Read the model definition and answer for the solid it produces. Units are mm, in the model's axes. A direction names the side the tool comes from. Coordinates: 2 decimals unless noted, no trailing zeros. Loops run counter-clockwise (first coordinate to the right, second up) from the corner with the lowest first, then second, coordinate; pieces in that order, holes last. Notation, with made-up numbers: (-14.5, 28.5) -> (16.5, 28.5) arc R28 cw to (16.5, 49.5) -> close; hole circle Ø9 at (54, 28). An arc over 180 degrees is marked (long way). Answer as a JSON object with one key per item and string values. Group by question number.
Q1. The part is cut by section B-B on x = 101.5. Write down the section's boundary in (y, z).
Q2. The part is cut by section A-A on y = 34. Write down the section's boundary in (x, z).
Q3. Each of these flat-tipped pins is pushed along its axis until it touches: P1, Ø2.5, axis at x = 83, y = 49, coming from the +Z side; P2, Ø1.5, axis at y = 2, z = 1.5, coming from the +X side; P3, Ø1.5, axis at y = 64, z = 1.5, coming from the +X side; P4, Ø0.9, axis at y = 14.5, z = 2, coming from the -X side. Where does it stop, or does it pass through?
Q4. Determine the mould class of faces 5 (the flat face through (76, 33, 3)), 6 (the flat face through (126, 13, 1)), 7 (the cylindrical face through (83.69, 47.67, 1.52)) for opening direction X: released by +X, released by -X, zero draft, split by the parting line, or undercut.
Q5. Straight lines are drawn through the part: line 1 along X through (y, z) = (36.5, 2); line 2 along Y through (x, z) = (114, 1.9); line 3 along X through (y, z) = (9, 2.8). For each, find the intervals that lie inside material, in ascending order. Write a range as [from, to].
Q6. For faces 1 (the flat face through (123, 33, 1)), 2 (the flat face through (123, 1, 1)), 3 (the flat face through (43, 64, 1)), 4 (the flat face through (99, 49, 2)), determine the directions among +Z, -Z, +X, -X, +Y, -Y from which every point of the face is accessible in a straight line to the end or side of a thin tool.
Q7. The part is cut by section C-C on y = 12.5. Write down the section's boundary in (x, z), and give its area (3 significant figures).
Q8. The part is cut by section D-D on z = 0.85. State how many separate pieces and enclosed holes the cut face has, and give its area (3 significant figures).
Autodesk Inventor part; units mm, degrees
ref_plane "YZ Plane" through (0, 0, 0) normal (1, 0, 0) x (0, 1, 0)
ref_plane "XZ Plane" through (0, 0, 0) normal (0, 1, 0) x (-1, 0, 0)
ref_plane "XY Plane" through (0, 0, 0) normal (0, 0, 1) x (1, 0, 0)
sketch "Sketch1" plane through (0, 0, 0) normal (0, 0, 1) x (1, 0, 0)
  line L0 (0, 0) -> (3, 0)
  line L1 (3, 0) -> (123, 0)
  line L2 (0, 0) -> (0, 3)
  line L3 (0, 3) -> (3, 3)
  line L4 (3, 3) -> (3, 23)
  line L5 (3, 23) -> (0, 23)
  line L6 (0, 23) -> (0, 43)
  line L7 (0, 43) -> (3, 43)
  line L8 (3, 43) -> (3, 63)
  line L9 (3, 63) -> (3, 66)
  line L10 (3, 66) -> (23, 66)
  line L11 (23, 66) -> (23, 63)
  line L12 (23, 63) -> (43, 63)
  line L13 (43, 63) -> (43, 66)
  line L14 (43, 66) -> (63, 66)
  line L15 (63, 66) -> (63, 63)
  line L16 (63, 63) -> (83, 63)
  line L17 (83, 63) -> (83, 66)
  line L18 (83, 66) -> (103, 66)
  line L19 (103, 66) -> (103, 63)
  line L20 (103, 63) -> (123, 63)
  line L21 (123, 63) -> (126, 63)
  line L22 (126, 63) -> (126, 43)
  line L23 (126, 43) -> (123, 43)
  line L24 (123, 43) -> (123, 23)
  line L25 (123, 23) -> (126, 23)
  line L26 (126, 23) -> (126, 3)
  line L27 (126, 3) -> (123, 3)
  line L28 (123, 0) -> (123, 3)
  dimension "d0" = 3
  dimension "d1" = 120
  dimension "d2" = 3
  dimension "d3" = 20
  dimension "d4" = 20
  dimension "d5" = 20
  dimension "d6" = 3
  dimension "d7" = 20
  dimension "d8" = 20
  dimension "d9" = 20
  dimension "d10" = 20
  dimension "d11" = 20
  dimension "d12" = 20
  dimension "d13" = 3
  dimension "d14" = 20
  dimension "d15" = 20
  dimension "d16" = 20
extrude "Extrusion1" add sketch "Sketch1" along normal blind 3
sketch "Sketch2" plane through (0, 0, 3) normal (0, 0, 1) x (1, 0, 0)
  line L0 (83, 49) -> (115, 49)
  line L1 (115, 49) -> (115, 17)
  line L2 (115, 17) -> (83, 17)
  line L3 (83, 17) -> (83, 49)
  line L4 (83, 49) -> (115, 17) construction
  line L5 (115, 49) -> (83, 17) construction
  line L6 (123, 23) -> (123, 43) construction
  circle A0 centre (83, 49) radius 1.5
  circle A1 centre (83, 17) radius 1.5
  circle A2 centre (115, 17) radius 1.5
  circle A3 centre (115, 49) radius 1.5
  line L7 (88.6569, 49) -> (83, 43.3431)
  line L8 (83, 22.6569) -> (88.6569, 17)
  line L9 (109.3431, 17) -> (115, 22.6569)
  line L10 (115, 43.3431) -> (109.3431, 49)
  point P0 (0, 0)
  point P1 (99, 33)
  point P2 (115, 33)
  point P3 (123, 33)
  dimension "d19" = 32
  dimension "d20" = 32
  dimension "d21" = 8
  dimension "d26" = 3
  dimension "d27" = 45
  dimension "d28" = 4
extrude "Extrusion2" cut sketch "Sketch2" against normal through all contours L3 A0 L0 | L0 A0 L3 | L0 L10 L1 L9 L2 L8 L3 L7 | A3 L1 L0 | L0 L1 A3 | A1 L2 L3 | L3 L2 A1 | A2 L2 L1 | L1 L2 A2
pattern_linear "Rectangular Pattern1" count 2 spacing 42 along (-1, 0, 0) of "Extrusion2"
sketch "Sketch3" plane through (0, 0, 3) normal (0, 0, 1) x (1, 0, 0)
  line L0 (8, 20) -> (28, 20)
  line L1 (28, 20) -> (28, 5)
  line L2 (28, 5) -> (8, 5)
  line L3 (8, 5) -> (8, 20)
  line L4 (0, 0) -> (123, 0)
  line L5 (3, 23) -> (3, 3)
  dimension "d34" = 15
  dimension "d35" = 5
  dimension "d36" = 5
  dimension "d37" = 20
extrude "Extrusion3" cut sketch "Sketch3" against normal through all
fillet "Fillet1" radius 4 4 edges at (28, 5, 1.5) (28, 20, 1.5) (8, 20, 1.5) (8, 5, 1.5)
properties part number "ControlBoxFace" material "Wood (Birch)"
Final values:
{
 "1": {"outline": "(0, 0) -> (17, 0) -> (17, 3) -> (0, 3) -> close; (49, 0) -> (66, 0) -> (66, 3) -> (49, 3) -> close"},
 "2": {"outline": "(0, 0) -> (41, 0) -> (41, 3) -> (0, 3) -> close; (73, 0) -> (83, 0) -> (83, 3) -> (73, 3) -> close; (115, 0) -> (123, 0) -> (123, 3) -> (115, 3) -> close"},
 "3": {"P1": "passes through", "P2": "stops at x = 123", "P3": "stops at x = 103", "P4": "stops at x = 3"},
 "4": {"face 5": "zero draft", "face 6": "released by +X", "face 7": "undercut"},
 "5": {"line 1": "x = [0, 41], [73, 83], [115, 123]", "line 2": "y = [0, 15.88], [18.12, 21.66], [44.34, 47.88], [50.12, 63]", "line 3": "x = [3, 8], [28, 126]"},
 "6": {"face 1": "+Z, -Z, +X", "face 2": "+Z, -Z, +X, -Y", "face 3": "+Z, -Z, +Y", "face 4": "+Z, -Z"},
 "7": {"outline": "(3, 0) -> (8, 0) -> (8, 3) -> (3, 3) -> close; (28, 0) -> (126, 0) -> (126, 3) -> (28, 3) -> close", "area": "309 mm2"},
 "8": {"separate pieces": "1", "enclosed holes": "11", "area": "5,670 mm2"}
}
